from build123d import *

# Parameters (mm, degrees)
BOSS_EXTRU_1_DEPTH      = 7
BOSS_EXTRU_1_DEPTH_BACK = 7
ESQUISSE1_R             = 35
ESQUISSE2_R             = 22
BOSS_EXTRU_2_DEPTH      = 2
BOSS_EXTRU_3_START      = 2
ESQUISSE3_R             = 22
BOSS_EXTRU_3_DEPTH      = 2
ESQUISSE4_R             = 14
BOSS_EXTRU_4_DEPTH      = 12
ESQUISSE5_R             = 3
ENL_V_MAT_EXTRU_1_DEPTH = 59


with BuildPart() as part:
    # Esquisse1 → Boss.-Extru.1 (new, two sides: drawn at the far end of the back side and taken through both)
    with BuildSketch(Plane.XY.offset(-BOSS_EXTRU_1_DEPTH_BACK)):
        Circle(ESQUISSE1_R)
    extrude(amount=BOSS_EXTRU_1_DEPTH + BOSS_EXTRU_1_DEPTH_BACK)

    # Esquisse2 → Boss.-Extru.2 (add)
    with BuildSketch(Plane.XY.offset(7)):
        Circle(ESQUISSE2_R)
    extrude(amount=BOSS_EXTRU_2_DEPTH)

    # Esquisse3 → Boss.-Extru.3 (add)
    with BuildSketch(Plane(origin=(0, 0, -7), x_dir=(-1, 0, 0), z_dir=(0, 0, -1)).offset(BOSS_EXTRU_3_START)):
        with Locations(Location((0, 0, 0), (0, 0, 180))):
            Circle(ESQUISSE3_R)
    extrude(amount=-BOSS_EXTRU_3_DEPTH)

    # Esquisse4 → Boss.-Extru.4 (add)
    with BuildSketch(Plane.XY.offset(9)):
        Circle(ESQUISSE4_R)
    extrude(amount=BOSS_EXTRU_4_DEPTH)

    # Esquisse5 → Enl_v. mat.-Extru.1 (cut)
    with BuildSketch(Plane(origin=(0, 0, -9), x_dir=(-1, 0, 0), z_dir=(0, 0, -1))):
        Circle(ESQUISSE5_R)
    extrude(amount=-ENL_V_MAT_EXTRU_1_DEPTH, mode=Mode.SUBTRACT)


solid = part.part
Geometry: final body of the model. Coordinates: model frame, mm. A direction names the side the tool comes from. Coordinates: 2 decimals unless noted, no trailing zeros. Order: outer loops, then holes, each group sorted by start corner. A loop starts at its lowest first (then second) coordinate and runs counter-clockwise, first axis right, second up.
(1) First-contact query: pin 1 (1 mm diameter, centred on y = 14, z = 0.5, fed in from +X); pin 2 (4 mm diameter, centred on y = -2, z = 14, fed in from +X); pin 3 (1.5 mm diameter, centred on x = -15.5, z = -4.5, fed in from -Y). Flat tips, straight axial feed; report the tip coordinate or a pass-through.
(2) Draft query along Y for faces 1 (the face through (-0.2, 3.3, 21)), 2 (the face through (3, 0, 6)), 3 (the face through (-4.769, -21.477, 7.986)). Return one class per face: pulls with the +Y half, pulls with the -Y half, needs draft (parallel to the pull), parting line crosses it, or undercut.
(3) Section query C-C (z = -2). Return the cut outline in (x, y), plus the area to 3 significant figures.
(4) Material intervals for probe 1 along Y at (x, z) = (0, 8); probe 2 along Y at (x, z) = (0, 1); probe 3 along Z at (x, y) = (27.5, -18.5), sorted ascending.
(5) Section query A-A (y = 0). Return the cut outline in (x, z).
(6) Section query D-D (x = 15.5). Return the cut outline in (y, z).
(7) Access query for faces 4 (the face through (0, -23, 7)), 5 (the face through (-4.769, 21.477, -8.014)), 6 (the face through (0, 5, -9)). Directions: +Z, -Z, +X, -X, +Y, -Y. A direction counts if a zero-diameter tool reaches every point of the face in a straight line with its end or side. Return the directions, or none.
Solution:
1. pin 1: stops at x = 32.29
1. pin 2: stops at x = 14
1. pin 3: stops at y = -31.74
2. face 1: needs draft
2. face 2: undercut
2. face 3: parting line crosses it
3. outline: circle Ø70 at (0, 0); hole circle Ø6 at (0, 0)
3. area: 3,820 mm2
4. probe 1: y = -22 to -3, 3 to 22
4. probe 2: y = -35 to -3, 3 to 35
4. probe 3: z = -7 to 7
5. outline: (-35, -7) - (-22, -7) - (-22, -9) - (-3, -9) - (-3, 21) - (-14, 21) - (-14, 9) - (-22, 9) - (-22, 7) - (-35, 7) - close; (3, -9) - (22, -9) - (22, -7) - (35, -7) - (35, 7) - (22, 7) - (22, 9) - (14, 9) - (14, 21) - (3, 21) - close
6. outline: (-31.38, -7) - (-15.61, -7) - (-15.61, -9) - (15.61, -9) - (15.61, -7) - (31.38, -7) - (31.38, 7) - (15.61, 7) - (15.61, 9) - (-15.61, 9) - (-15.61, 7) - (-31.38, 7) - close
7. face 4: +Z
7. face 5: -Z
7. face 6: -Z, +X, -X, +Y, -Y
